```python
from build123d import *

# Parameters (mm, degrees)
SKETCH005_R             = 1.55
PAD_DEPTH               = 1.6
SKETCH016_W             = 1.994334
SKETCH016_H             = 1.107967
SKETCH016_W_2           = 3.619357
SKETCH016_H_2           = 1.255696
SKETCH016_H_3           = 1.551151
SKETCH016_W_3           = 2.732976
SKETCH016_H_4           = 1.403424
SKETCH016_W_4           = 2.880716
SKETCH016_H_5           = 1.181828
SKETCH016_W_5           = 1.625016
SKETCH016_H_6           = 2.51139
SKETCH016_W_6           = 0.960235
SKETCH016_H_7           = 3.47163
SKETCH016_W_7           = 1.994338
SKETCH016_H_8           = 3.323896
SKETCH016_W_8           = 1.107967
SKETCH016_H_9           = 3.176168
SKETCH016_W_9           = 3.693223
SKETCH016_H_10          = 1.477287
SKETCH016_W_10          = 4.13641
SKETCH016_H_11          = 1.625017
SKETCH016_W_11          = 3.76297
SKETCH016_H_12          = 1.485384
SKETCH016_W_12          = 1.395884
SKETCH016_H_13          = 3.115539
SKETCH016_W_13          = 1.446203
SKETCH016_H_14          = 2.63131
SKETCH016_W_14          = 1.448886
SKETCH016_H_15          = 3.323898
SKETCH016_W_15          = 1.772745
SKETCH016_H_16          = 2.215931
SKETCH016_W_16          = 1.625013
SKETCH016_H_17          = 2.707825
SKETCH016_W_17          = 1.312852
SKETCH016_H_18          = 3.187283
SKETCH016_W_18          = 1.846609
SKETCH016_H_19          = 2.954575
SKETCH016_W_19          = 1.551152
SKETCH016_H_20          = 2.46188
SKETCH016_W_20          = 4.159074
SKETCH016_H_21          = 3.862
SKETCH016_R             = 0.720914
SKETCH016_W_21          = 5
SKETCH016_H_22          = 5
SKETCH016_R_2           = 0.816015
PAD004_DEPTH            = 2
PAD007_DEPTH            = 1.6
BODY002_PLACEMENT_ANGLE = 180


with BuildPart() as part:
    # Sketch005 → Pad (new body)
    with BuildSketch(Plane.XY):
        with BuildLine():
            Line((-35, 92), (35, 92))
            Line((35, 92), (35, 12))
            ThreePointArc((23, 0), (31.485281, 3.514719), (35, 12))
            Line((23, 0), (-23, 0))
            ThreePointArc((-35, 12), (-31.485281, 3.514719), (-23, 0))
            Line((-35, 12), (-35, 92))
        make_face()
        with Locations((-23, 60)):
            Circle(SKETCH005_R, mode=Mode.SUBTRACT)
        with Locations((29, 56)):
            Circle(SKETCH005_R, mode=Mode.SUBTRACT)
        with Locations((29, 20)):
            Circle(SKETCH005_R, mode=Mode.SUBTRACT)
        with Locations((20, 5)):
            Circle(SKETCH005_R, mode=Mode.SUBTRACT)
        with Locations((-20, 5)):
            Circle(SKETCH005_R, mode=Mode.SUBTRACT)
        with BuildLine():
            Line((-2.5, 54.5), (-16.5, 54.5))
            Line((-16.5, 54.5), (-16.5, 40.5))
            ThreePointArc((-17.5, 40.5), (-17, 40), (-16.5, 40.5))
            Line((-17.5, 40.5), (-17.5, 54.5))
            ThreePointArc((-16.5, 55.5), (-17.207107, 55.207107), (-17.5, 54.5))
            Line((-16.5, 55.5), (-2.5, 55.5))
            ThreePointArc((-2.5, 54.5), (-2, 55), (-2.5, 55.5))
        make_face(mode=Mode.SUBTRACT)
        with BuildLine():
            Line((2.5, 21.5), (16.5, 21.5))
            Line((16.5, 21.5), (16.5, 35.5))
            ThreePointArc((17.5, 35.5), (17, 36), (16.5, 35.5))
            Line((17.5, 35.5), (17.5, 21.5))
            ThreePointArc((16.5, 20.5), (17.207107, 20.792893), (17.5, 21.5))
            Line((16.5, 20.5), (2.5, 20.5))
            ThreePointArc((2.5, 21.5), (2, 21), (2.5, 20.5))
        make_face(mode=Mode.SUBTRACT)
        with BuildLine():
            Line((2.5, 54.5), (16.5, 54.5))
            Line((16.5, 40.5), (16.5, 54.5))
            ThreePointArc((16.5, 40.5), (17, 40), (17.5, 40.5))
            Line((17.5, 54.5), (17.5, 40.5))
            ThreePointArc((17.5, 54.5), (17.207107, 55.207107), (16.5, 55.5))
            Line((16.5, 55.5), (2.5, 55.5))
            ThreePointArc((2.5, 55.5), (2, 55), (2.5, 54.5))
        make_face(mode=Mode.SUBTRACT)
        with BuildLine():
            Line((-2.5, 21.5), (-16.5, 21.5))
            Line((-16.5, 35.5), (-16.5, 21.5))
            ThreePointArc((-16.5, 35.5), (-17, 36), (-17.5, 35.5))
            Line((-17.5, 21.5), (-17.5, 35.5))
            ThreePointArc((-17.5, 21.5), (-17.207107, 20.792893), (-16.5, 20.5))
            Line((-16.5, 20.5), (-2.5, 20.5))
            ThreePointArc((-2.5, 20.5), (-2, 21), (-2.5, 21.5))
        make_face(mode=Mode.SUBTRACT)
        with BuildLine():
            Line((-13, 59.5), (13, 59.5))
            ThreePointArc((13, 58.5), (13.5, 59), (13, 59.5))
            Line((-13, 58.5), (13, 58.5))
            ThreePointArc((-13, 59.5), (-13.5, 59), (-13, 58.5))
        make_face(mode=Mode.SUBTRACT)
        with BuildLine():
            Line((13, 16.5), (-13, 16.5))
            ThreePointArc((-13, 17.5), (-13.5, 17), (-13, 16.5))
            Line((13, 17.5), (-13, 17.5))
            ThreePointArc((13, 16.5), (13.5, 17), (13, 17.5))
        make_face(mode=Mode.SUBTRACT)
        with BuildLine():
            Line((-21.5, 51), (-21.5, 25))
            ThreePointArc((-21.5, 25), (-21, 24.5), (-20.5, 25))
            Line((-20.5, 51), (-20.5, 25))
            ThreePointArc((-20.5, 51), (-21, 51.5), (-21.5, 51))
        make_face(mode=Mode.SUBTRACT)
        with BuildLine():
            Line((21.5, 25), (21.5, 51))
            ThreePointArc((21.5, 51), (21, 51.5), (20.5, 51))
            Line((20.5, 25), (20.5, 51))
            ThreePointArc((20.5, 25), (21, 24.5), (21.5, 25))
        make_face(mode=Mode.SUBTRACT)
    extrude(amount=PAD_DEPTH)

    # Sketch016 → Pad004 (join)
    with BuildSketch(Plane.XY.offset(-1.5)):
        with Locations((-10.621927, 50.160947)):
            Rectangle(SKETCH016_W, SKETCH016_H)
        with Locations((-5.820745, 49.939356)):
            Rectangle(SKETCH016_W_2, SKETCH016_H_2)
        with Locations((-0.20705, 50.160947)):
            Rectangle(SKETCH016_W_2, SKETCH016_H_3)
        with Locations((5.480506, 49.71776)):
            Rectangle(SKETCH016_W_3, SKETCH016_H_4)
        with Locations((10.872605, 49.902422)):
            Rectangle(SKETCH016_W_4, SKETCH016_H_5)
        with Locations((11.722045, 45.544422)):
            Rectangle(SKETCH016_W_5, SKETCH016_H_6)
        with Locations((11.980572, 39.672205)):
            Rectangle(SKETCH016_W_6, SKETCH016_H_7)
        with Locations((12.276028, 32.950547)):
            Rectangle(SKETCH016_W_7, SKETCH016_H_8)
        with Locations((12.497625, 27.484584)):
            Rectangle(SKETCH016_W_8, SKETCH016_H_9)
        with Locations((6.994723, 26.487413)):
            Rectangle(SKETCH016_W_9, SKETCH016_H_10)
        with Locations((-0.613303, 26.487414)):
            Rectangle(SKETCH016_W_10, SKETCH016_H_11)
        with Locations((-9.603089, 26.466649)):
            Rectangle(SKETCH016_W_11, SKETCH016_H_12)
        with Locations((-11.142747, 31.147487)):
            Rectangle(SKETCH016_W_12, SKETCH016_H_13)
        with Locations((-10.969857, 36.694603)):
            Rectangle(SKETCH016_W_13, SKETCH016_H_14)
        with Locations((-10.894651, 42.061836)):
            Rectangle(SKETCH016_W_14, SKETCH016_H_15)
        with Locations((-10.215674, 46.13534)):
            Rectangle(SKETCH016_W_15, SKETCH016_H_16)
        with Locations((4.805575, 44.245694)):
            Rectangle(SKETCH016_W_16, SKETCH016_H_17)
        with Locations((5.287496, 34.348413)):
            Rectangle(SKETCH016_W_17, SKETCH016_H_18)
        with Locations((-2.940033, 33.873852)):
            Rectangle(SKETCH016_W_18, SKETCH016_H_19)
        with Locations((-3.112926, 44.121912)):
            Rectangle(SKETCH016_W_19, SKETCH016_H_20)
        with Locations((0.745081, 39.092407)):
            Rectangle(SKETCH016_W_20, SKETCH016_H_21)
        with Locations((0.844105, 39.141918)):
            Circle(SKETCH016_R, mode=Mode.SUBTRACT)
        with Locations((0.024826, 64.643266)):
            Rectangle(SKETCH016_W_21, SKETCH016_H_22)
        with Locations((0, 64.519768)):
            Circle(SKETCH016_R_2, mode=Mode.SUBTRACT)
    extrude(amount=PAD004_DEPTH)

    # Sketch023 → Pad007 (join)
    with BuildSketch(Plane.XY):
        with BuildLine():
            Line((-12.85, 0), (12.85, 0))
            Line((12.85, 0), (12.85, -11.654535))
            ThreePointArc((7.85, -16.654535), (11.385534, -15.190069), (12.85, -11.654535))
            Line((7.85, -16.654535), (-7.85, -16.654535))
            ThreePointArc((-12.85, -11.654535), (-11.385534, -15.190069), (-7.85, -16.654535))
            Line((-12.85, -11.654535), (-12.85, 0))
        make_face()
    extrude(amount=PAD007_DEPTH)


with BuildPart() as part_1:
    # Body002 placement: moved
    add(part.part.rotate(Axis((0, 0, 0), (0, 1, 0)), BODY002_PLACEMENT_ANGLE))


solid = part_1.part
```
Geometry check sheet. Reference: the model listing, model coordinates, mm. Give positions to 0.01 mm unless a question says otherwise; leave off trailing zeros. Write each loop counter-clockwise with the first axis right and the second up, starting at its lowest first coordinate (ties: lowest second). Pieces come first, ordered by that corner, then holes.
1) Material ranges on L1, parallel to Y at x = 0, z = 0.4; L2, parallel to X at y = 52, z = -0.5; L3, parallel to Y at x = -20, z = -0.8, recorded low to high.
2) Release check for a two-part mould opening along X. For faces 1 (the cylindrical face through (23.202, 61.537, -0.789)), 2 (the flat face through (1, 65, 1.5)), 3 (the cylindrical face through (31.58, 3.61, -0.79)) record: pulls with the +X half, pulls with the -X half, needs draft (parallel to the pull), parting line crosses it, or undercut.
3) Section check B-B, the plane z = -1. State how many separate pieces and enclosed holes the cut face has, and give its area (3 significant figures).
4) Section check A-A, the plane x = -29.5. Record the boundary of the cut face in (y, z).
5) Section check C-C, the plane y = 73. Record the boundary of the cut face in (x, z), and give its area (3 significant figures).
6) Gauge pin test, flat ends, axial feed: pin 1 (0.7 mm diameter, centred on y = 49.5, z = 1, fed in from -X); pin 2 (0.5 mm diameter, centred on x = 10.5, z = 1, fed in from -Y); pin 3 (1.7 mm diameter, centred on x = -11, z = 1, fed in from -Y). Record the tip position at first contact, or that the pin passes through.
7) Section check D-D, the plane x = 31. Record the boundary of the cut face in (y, z), and give its area (3 significant figures).
Computed:
1. L1: y = 25.67 to 27.3, 37.16 to 41.02, 49.39 to 50.94, 62.14 to 63.7, 65.34 to 67.14
1. L2: x = -35 to -17.5, -16.5 to 16.5, 17.5 to 35
1. L3: y = 0 to 3.45, 6.55 to 92
2. face 1: undercut
2. face 2: needs draft
2. face 3: pulls with the +X half
3. separate pieces: 1
3. enclosed holes: 13
3. area: 6,530 mm2
4. outline: (1.91, -1.6) - (18.53, -1.6) - (18.53, 0) - (1.91, 0) - close; (21.47, -1.6) - (54.53, -1.6) - (54.53, 0) - (21.47, 0) - close; (57.47, -1.6) - (92, -1.6) - (92, 0) - (57.47, 0) - close
5. outline: (-35, -1.6) - (35, -1.6) - (35, 0) - (-35, 0) - close
5. area: 112 mm2
6. pin 1: stops at x = -12.31
6. pin 2: stops at y = 25.72
6. pin 3: stops at y = 31.29
7. outline: (3.06, -1.6) - (92, -1.6) - (92, 0) - (3.06, 0) - close
7. area: 142 mm2
